Read the model definition and answer for the solid it produces. Units are mm, in the model's axes. Coordinates: 2 decimals unless noted, no trailing zeros. Write each loop counter-clockwise with the first axis right and the second up, starting at its lowest first coordinate (ties: lowest second). Pieces come first, ordered by that corner, then holes.
(1) Find the intervals of material crossed by probe 1 along Y at (x, z) = (3.1, 15); probe 2 along Z at (x, y) = (5.5, 5); probe 3 along X at (y, z) = (6, 248), in increasing order.
(2) Section A-A on z = 109 is taken. Write down the section's boundary in (x, y), then the cut area to 3 significant figures.
(3) Given pin 1 (3 mm diameter, centred on y = 6.05, z = 385, fed in from +X); pin 2 (5 mm diameter, centred on y = 6.5, z = 119.5, fed in from -X), each flat-ended and moving along its own axis, determine where each tip first touches the part or whether it passes through.
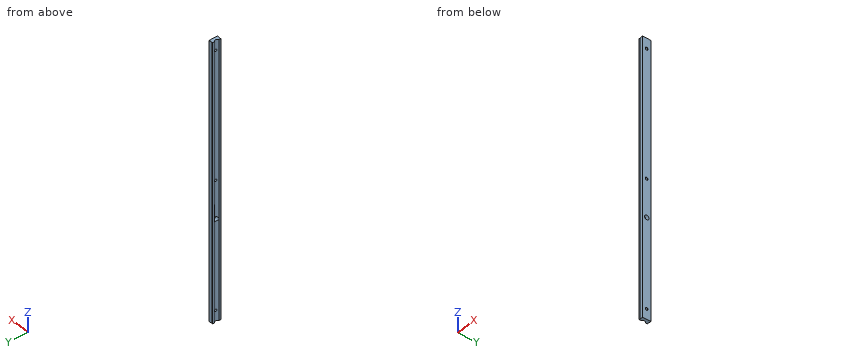
from build123d import *

# Parameters (mm, degrees)
BOSS_EXTRUDE1_DEPTH = 400
SKETCH5_R           = 3.25
CUT_EXTRUDE1_DEPTH  = 6


with BuildPart() as part:
    # Sketch1 → Boss-Extrude1 (new body)
    with BuildSketch(Plane.XY):
        with BuildLine():
            Line((0, 2.974695), (0, 0))
            Line((0, 0), (0.305573, 0))
            ThreePointArc((0.305573, 0), (1.2, 0.4), (2.094427, 0))
            Line((2.094427, 0), (5.8, 0))
            Line((5.8, 0), (5.8, 12.1))
            Line((5.8, 12.1), (2.094427, 12.1))
            ThreePointArc((2.094427, 12.1), (1.2, 11.7), (0.305573, 12.1))
            Line((0.305573, 12.1), (0, 12.1))
            Line((0, 12.1), (0, 9.125305))
            ThreePointArc((0, 9.125305), (1.95, 6.05), (0, 2.974695))
        make_face()
    extrude(amount=BOSS_EXTRUDE1_DEPTH)

    # Sketch2 → Cut-Revolve1 (revolve, cut)
    with BuildSketch(Plane.XY.offset(15)):
        Polygon((1.299545, 6.05), (1.299545, 8.05), (1.678545, 7.671), (5.421, 7.671), (5.8, 8.05), (5.8, 6.05), align=None)
    revolve(axis=Axis((5.8, 6.05, 15), (-1, 0, 0)), mode=Mode.SUBTRACT)

    # Sketch3 → Cut-Revolve2 (revolve, cut)
    with BuildSketch(Plane.XY.offset(385)):
        Polygon((1.299545, 6.05), (1.299545, 8.05), (1.678545, 7.671), (5.421, 7.671), (5.8, 8.05), (5.8, 6.05), align=None)
    revolve(axis=Axis((5.8, 6.05, 385), (-1, 0, 0)), mode=Mode.SUBTRACT)

    # Sketch4 → Cut-Revolve3 (revolve, cut)
    with BuildSketch(Plane.XY.offset(200)):
        Polygon((1.299545, 6.05), (1.299545, 8.05), (1.678545, 7.671), (5.421, 7.671), (5.8, 8.05), (5.8, 6.05), align=None)
    revolve(axis=Axis((5.8, 6.05, 200), (-1, 0, 0)), mode=Mode.SUBTRACT)

    # Sketch5 → Cut-Extrude1 (cut)
    with BuildSketch(Plane(origin=(5.8, 0, 0), x_dir=(0, 0, -1), z_dir=(1, 0, 0))):
        with Locations((-145, 6.05)):
            Circle(SKETCH5_R)
    extrude(amount=-CUT_EXTRUDE1_DEPTH, mode=Mode.SUBTRACT)


solid = part.part
Response:
1. probe 1: y = 0 to 4.43, 7.67 to 12.1
1. probe 2: z = 0 to 13.66, 16.34 to 141.92, 148.08 to 198.66, 201.34 to 383.66, 386.34 to 400
1. probe 3: x = 1.95 to 5.8
2. outline: (0, 0) - (0.31, 0) arc R1.2 cw to (2.09, 0) - (5.8, 0) - (5.8, 12.1) - (2.09, 12.1) arc R1.2 cw to (0.31, 12.1) - (0, 12.1) - (0, 9.13) arc R3.4 cw to (0, 2.97) - close
2. area: 60.6 mm2
3. pin 1: passes through
3. pin 2: stops at x = 0.24
